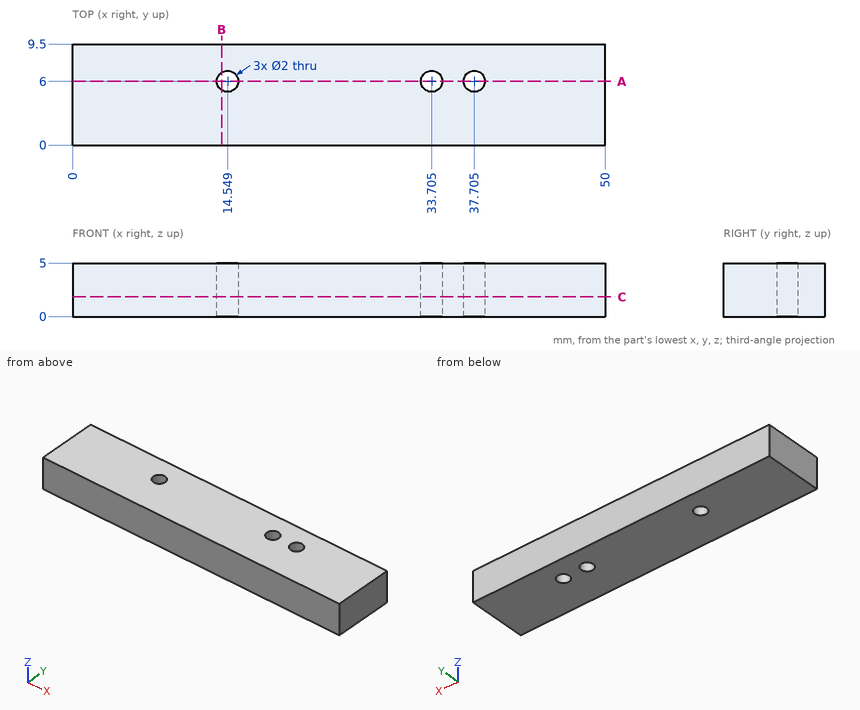
Design review of the part shown in the three views and the two pictorial views. Dimensions are in mm from the part's minimum x, y and z. Round coordinates to 2 decimals unless told otherwise and drop trailing zeros. Loops run counter-clockwise (first coordinate to the right, second up) from the corner with the lowest first, then second, coordinate; pieces in that order, holes last.
Q1. To check wall thickness, follow line 1 along X through (y, z) = (5.5, 3.6) (1 decimal); line 2 along Y through (x, z) = (37, 3.35). State the ranges of each line that lie inside material, in increasing order.
Result sheet:
line 1: x = 0 to 13.7, 15.4 to 32.8, 34.6 to 36.8, 38.6 to 50
line 2: y = 0 to 5.29, 6.71 to 9.5
Q2. Add section A-A on y = 6. Write out the cut boundary in (x, z) (1 decimal).
Result sheet:
outline: (0, 0) - (13.5, 0) - (13.5, 5) - (0, 5) - close; (15.5, 0) - (32.7, 0) - (32.7, 5) - (15.5, 5) - close; (34.7, 0) - (36.7, 0) - (36.7, 5) - (34.7, 5) - close; (38.7, 0) - (50, 0) - (50, 5) - (38.7, 5) - close
Q3. Add section B-B on x = 14. Write out the cut boundary in (y, z).
Result sheet:
outline: (0, 0) - (5.16, 0) - (5.16, 5) - (0, 5) - close; (6.84, 0) - (9.5, 0) - (9.5, 5) - (6.84, 5) - close
Q4. Add section C-C on z = 1.85. Write out the cut boundary in (x, y) (1 decimal).
Result sheet:
outline: (0, 0) - (50, 0) - (50, 9.5) - (0, 9.5) - close; hole circle Ø2 at (14.5, 6); hole circle Ø2 at (33.7, 6); hole circle Ø2 at (37.7, 6)
